```python
from build123d import *

# Parameters (mm, degrees)
F0_W     = 433
F0_H     = 293
F1_DEPTH = 116
F2_T     = -4
F4_D     = 21
F4_DEPTH = 5


with BuildPart() as f1:
    # F0 (on Top) → F1 (new body)
    with BuildSketch(Plane.XY):
        Rectangle(F0_W, F0_H)
    extrude(amount=F1_DEPTH)

    # F2
    f2_openings = [f1.faces().sort_by_distance(p)[0] for p in [
        (0, 0, 116),
    ]]
    offset(amount=F2_T, openings=f2_openings)

    # F4
    with Locations(Plane(origin=(-216.5, 0, 0), x_dir=(0, -1, 0), z_dir=(-1, 0, 0))):
        with Locations((0, 40)):
            Hole(F4_D / 2, depth=F4_DEPTH)


solid = f1.part
```
Input: part model. Units: mm. Frame: model coordinates. A direction names the side the tool comes from. Coordinates: 2 decimals unless noted, no trailing zeros. Loops run counter-clockwise (first coordinate to the right, second up) from the corner with the lowest first, then second, coordinate; pieces in that order, holes last.
Q1. Mould query, pull axis Y, two halves, no side actions, for faces 4 (the flat face through (-3, 146.5, 57)), 5 (the flat face through (-3, -142.5, 59)), 6 (the flat face through (216.5, -2, 57)), 7 (the flat face through (-3, 142.5, 59)). Classes: +Y half, -Y half, draft (parallel to the pull), parting line (faces both ways), or undercut.
Results are:
face 4: +Y half
face 5: undercut
face 6: draft
face 7: undercut
Q2. Section B-B, the plane z = 79.5. Return the cut outline in (x, y).
Results are:
outline: (-216.5, -146.5) - (216.5, -146.5) - (216.5, 146.5) - (-216.5, 146.5) - close; hole (-212.5, -142.5) - (212.5, -142.5) - (212.5, 142.5) - (-212.5, 142.5) - close
Q3. Set-up query: faces 1 (the flat face through (-212.5, -2, 59)), 2 (the cylindrical face through (-214.472, 4.845, 30.685)), 3 (the flat face through (-216.5, -2, 57)). Return all of +Z, -Z, +X, -X, +Y, -Y with unobstructed straight access to the full face (end or side cutting, diameter ignored); none if empty.
Results are:
face 1: +Z
face 2: -X
face 3: +Z, -Z, -X, +Y, -Y
Q4. Line query: line 1 along X through (y, z) = (123, 83); line 2 along Z through (x, y) = (-214.9, 0); line 3 along Y through (x, z) = (199.5, 32.5). Output: solid intervals per line, ascending.
Results are:
line 1: x = -216.5 to -212.5, 212.5 to 216.5
line 2: z = 0 to 29.5, 50.5 to 116
line 3: y = -146.5 to -142.5, 142.5 to 146.5
Q5. Section A-A, the plane y = 0. Return the cut outline in (x, z), and give its area (3 significant figures).
Results are:
outline: (-216.5, 0) - (216.5, 0) - (216.5, 116) - (212.5, 116) - (212.5, 4) - (-212.5, 4) - (-212.5, 29.5) - (-216.5, 29.5) - close; (-216.5, 50.5) - (-212.5, 50.5) - (-212.5, 116) - (-216.5, 116) - close
area: 2,540 mm2
Q6. Section D-D, the plane y = -42. Return the cut outline in (x, z), and give its area (3 significant figures).
Results are:
outline: (-216.5, 0) - (216.5, 0) - (216.5, 116) - (212.5, 116) - (212.5, 4) - (-212.5, 4) - (-212.5, 116) - (-216.5, 116) - close
area: 2,630 mm2
Q7. Contact query for flat-ended pins moving along their axis: pin 1 (12 mm diameter, centred on x = -17, y = -48.5, fed in from -Z); pin 2 (1.5 mm diameter, centred on x = 48, y = 111.5, fed in from +Z). Output: stop coordinate, or through.
Results are:
pin 1: stops at z = 0
pin 2: stops at z = 4
Q8. Section C-C, the plane x = -139. Return the cut outline in (y, z), and give its area (3 significant figures).
Results are:
outline: (-146.5, 0) - (146.5, 0) - (146.5, 116) - (142.5, 116) - (142.5, 4) - (-142.5, 4) - (-142.5, 116) - (-146.5, 116) - close
area: 2,070 mm2
